```python
from build123d import *

# Parameters (mm, degrees)
ESQUISSE1_R               = 1
BOSS_EXTRU_2_DEPTH        = 6
ESQUISSE5_R               = 2
ENL_V_MAT_EXTRU_1_DEPTH   = 2
SYM_TRIE2_COPY_1_SKETCH_R = 2
SYM_TRIE2_COPY_1_DEPTH    = 2


with BuildPart() as part:
    # Esquisse1 → Boss.-Extru.2 (new body)
    with BuildSketch(Plane.XY):
        with BuildLine():
            Line((-8.804987496, 15.007737844), (-7.539903085, 12.851453671))
            ThreePointArc((-7.539903085, 12.851453671), (-5.096100136, 14.00142005), (-2.484854326, 14.691340952))
            Line((-2.484854326, 14.691340952), (-2.901776193, 17.156331045))
            ThreePointArc((-2.901776193, 17.156331045), (0, 17.4), (2.901776193, 17.156331045))
            Line((2.901776193, 17.156331045), (2.484854326, 14.691340952))
            ThreePointArc((2.484854326, 14.691340952), (5.096100136, 14.00142005), (7.539903085, 12.851453671))
            Line((7.539903085, 12.851453671), (8.804987496, 15.007737844))
            ThreePointArc((8.804987496, 15.007737844), (11.184504409, 13.32917331), (13.250766551, 11.277286278))
            Line((13.250766551, 11.277286278), (11.346920782, 9.656986526))
            ThreePointArc((11.346920782, 9.656986526), (12.903778516, 7.45), (14.036656047, 4.998228389))
            Line((14.036656047, 4.998228389), (16.391799678, 5.836857314))
            ThreePointArc((16.391799678, 5.836857314), (17.135654902, 3.021478291), (17.399575974, 0.121473929))
            Line((17.399575974, 0.121473929), (14.899636898, 0.104020778))
            ThreePointArc((14.899636898, 0.104020778), (14.67363552, -2.587357847), (13.965501643, -5.193723505))
            Line((13.965501643, -5.193723505), (16.308706617, -6.065153623))
            ThreePointArc((16.308706617, -6.065153623), (15.068842026, -8.7), (13.406930424, -11.091177422))
            Line((13.406930424, -11.091177422), (11.480647317, -9.497617447))
            ThreePointArc((11.480647317, -9.497617447), (9.577535384, -11.414062202), (7.359733812, -12.95547445))
            Line((7.359733812, -12.95547445), (8.594588479, -15.129211773))
            ThreePointArc((8.594588479, -15.129211773), (5.951150494, -16.350651602), (3.141033127, -17.114143592))
            Line((3.141033127, -17.114143592), (2.689735264, -14.655214915))
            ThreePointArc((2.689735264, -14.655214915), (0, -14.9), (-2.689735264, -14.655214915))
            Line((-2.689735264, -14.655214915), (-3.141033127, -17.114143592))
            ThreePointArc((-3.141033127, -17.114143592), (-5.951150494, -16.350651602), (-8.594588479, -15.129211773))
            Line((-8.594588479, -15.129211773), (-7.359733812, -12.95547445))
            ThreePointArc((-7.359733812, -12.95547445), (-9.577535384, -11.414062202), (-11.480647317, -9.497617447))
            Line((-11.480647317, -9.497617447), (-13.406930424, -11.091177422))
            ThreePointArc((-13.406930424, -11.091177422), (-15.068842026, -8.7), (-16.308706617, -6.065153623))
            Line((-16.308706617, -6.065153623), (-13.965501643, -5.193723505))
            ThreePointArc((-13.965501643, -5.193723505), (-14.67363552, -2.587357847), (-14.899636898, 0.104020778))
            Line((-14.899636898, 0.104020778), (-17.399575974, 0.121473929))
            ThreePointArc((-17.399575974, 0.121473929), (-17.135654902, 3.021478291), (-16.391799678, 5.836857314))
            Line((-16.391799678, 5.836857314), (-14.036656047, 4.998228389))
            ThreePointArc((-14.036656047, 4.998228389), (-12.903778516, 7.45), (-11.346920782, 9.656986526))
            Line((-11.346920782, 9.656986526), (-13.250766551, 11.277286278))
            ThreePointArc((-13.250766551, 11.277286278), (-11.184504409, 13.32917331), (-8.804987496, 15.007737844))
        make_face()
        with Locations((-6.5, -8.25)):
            Circle(ESQUISSE1_R, mode=Mode.SUBTRACT)
        with Locations((-6.5, 8.25)):
            Circle(ESQUISSE1_R, mode=Mode.SUBTRACT)
        with Locations((6.5, -8.25)):
            Circle(ESQUISSE1_R, mode=Mode.SUBTRACT)
        with Locations((6.5, 8.25)):
            Circle(ESQUISSE1_R, mode=Mode.SUBTRACT)
    extrude(amount=BOSS_EXTRU_2_DEPTH)

    # Esquisse3 → Révolution1 (revolve)
    with BuildSketch(Plane(origin=(0, 0, 0), x_dir=(1, 0, 0), z_dir=(0, 1, 0))):
        Polygon((0, -6), (-5.5, -6), (-5.5, -6.4), (-4.965, -6.4), (-4.965, -10.4), (0, -10.4), align=None)
    revolve(axis=Axis((0, 0, -3.652866049), (0, 0, 1)))

    # Esquisse4 → Enlèvement de matière-Révolution1 (revolve, cut)
    with BuildSketch(Plane(origin=(0, 0, 0), x_dir=(1, 0, 0), z_dir=(0, 1, 0)), mode=Mode.PRIVATE) as enl_vement_de_mati_re_r_volution1_sk:
        Polygon((-2.65, -6.72), (-2.65, -8.4), (-4, -8.4), (-4, -10.4), (0, -10.4), (0, 0), (-12.6, 0), (-12.6, -2.5), (-8, -2.5), (-8, -4.72), (-4, -4.72), (-4, -6.72), align=None)
    revolve(enl_vement_de_mati_re_r_volution1_sk.sketch.rotate(Axis((0, 0, 13.157502932), (0, 0, -1)), 180), axis=Axis((0, 0, 13.157502932), (0, 0, -1)), mode=Mode.SUBTRACT)

    # Esquisse5 → Enlèv. mat.-Extru.1 (cut)
    with BuildSketch(Plane.XY.offset(6)):
        with Locations((-6.5, 8.25)):
            Circle(ESQUISSE5_R)
    enl_v_mat_extru_1 = extrude(amount=-ENL_V_MAT_EXTRU_1_DEPTH, mode=Mode.SUBTRACT)

    # Symétrie1: Enlèv. mat.-Extru.1 across plane
    add(enl_v_mat_extru_1.mirror(Plane.ZX), mode=Mode.SUBTRACT)

    # Symétrie2: Enlèv. mat.-Extru.1 across plane
    add(enl_v_mat_extru_1.mirror(Plane(origin=(0, 0, 0), x_dir=(0, 0, 1), z_dir=(1, 0, 0))), mode=Mode.SUBTRACT)

    # Symétrie2 copy 1 sketch → Symétrie2 copy 1 (cut)
    with BuildSketch(Plane(origin=(0, 0, 6), x_dir=(-1, 0, 0), z_dir=(0, 0, 1))):
        with Locations((-6.5, 8.25)):
            Circle(SYM_TRIE2_COPY_1_SKETCH_R)
    extrude(amount=-SYM_TRIE2_COPY_1_DEPTH, mode=Mode.SUBTRACT)


solid = part.part
```
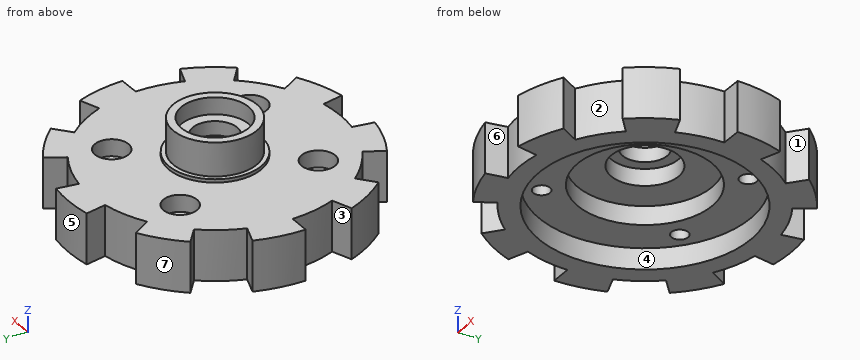
For this review, take the finished solid that the model builds, in its own axes (mm). Face numbers are marked on the shaded views. A direction names the side the tool comes from. Coordinates: 2 decimals unless noted, no trailing zeros. Order: outer loops, then holes, each group sorted by start corner. A loop starts at its lowest first (then second) coordinate and runs counter-clockwise, first axis right, second up. Notation, with made-up numbers: (-16.75, 14) - (28.25, 14) arc R20 ccw to (28.25, 22) - close; hole circle Ø2 at (13, 18.25). An arc over 180 degrees is marked (long way). Answer as a JSON object with one key per item and string values. Group by question number.
1. We need section D-D on z = 7.75. State the section outline as (x, y) points (3 decimals).
2. Clearance check with flat-ended pins moving along their axes: P1, Ø2, axis at y = 9.5, z = 7.5, coming from the -X side; P2, Ø9, axis at x = 0, y = 0, coming from the +Z side; P3, Ø3, axis at x = 7.5, y = 7.5, coming from the +Z side; P4, Ø1.2, axis at x = -6.5, y = 9, coming from the +Z side. State where each tip first meets the part, or that it passes through.
3. The part is to be moulded in two halves that separate along X. For the marked faces 5, 6 and 7, say which applies: pulls with the +X half, pulls with the -X half, needs draft (parallel to the pull), parting line crosses it, or undercut.
4. We need section C-C on z = 3.25. Give the number of separate pieces and of enclosed holes in the cut face, then the cut area to 3 significant figures.
5. For the marked faces 1, 2, 3 and 4, list the 3-axis set-ups (+Z, -Z, +X, -X, +Y, -Y) from which the entire face can be reached by the end or side of a thin tool; tool diameter is ignored.
6. We need section B-B on x = -6.5. State the section outline as (y, z) points, then the cut area to 3 significant figures.
7. For probe 1 along X at (y, z) = (8.25, 3.3); probe 2 along Y at (x, z) = (-6.5, 3.2); probe 3 along Y at (x, z) = (13, 5.5), list the stretches that pass through material, from the lowest coordinate up.
Final values:
{
 "1": {"outline": "circle Ø9.93 at (0, 0); hole circle Ø5.3 at (0, 0)"},
 "2": {"P1": "through", "P2": "z = 10.4", "P3": "z = 6", "P4": "z = 4"},
 "3": {"face 5": "parting line crosses it", "face 6": "undercut", "face 7": "pulls with the -X half"},
 "4": {"separate pieces": "1", "enclosed holes": "5", "area": "606 mm²"},
 "5": {"face 1": "+Z, -Z, +X", "face 2": "+Z, -Z", "face 3": "+Z, -Z, -X", "face 4": "-Z"},
 "6": {"outline": "(-16.14, 0) - (-10.79, 0) - (-10.79, 2.5) - (-9.25, 2.5) - (-9.25, 4) - (-10.25, 4) - (-10.25, 6) - (-16.14, 6) - close; (-7.25, 2.5) - (-4.66, 2.5) - (-4.66, 4.72) - (4.66, 4.72) - (4.66, 2.5) - (7.25, 2.5) - (7.25, 4) - (6.25, 4) - (6.25, 6) - (-6.25, 6) - (-6.25, 4) - (-7.25, 4) - close; (9.25, 2.5) - (10.79, 2.5) - (10.79, 0) - (13.41, 0) - (13.41, 6) - (10.25, 6) - (10.25, 4) - (9.25, 4) - close", "area": "80.6 mm²"},
 "7": {"probe 1": "-12.41 to -7.5, -5.5 to 5.5, 7.5 to 12.41", "probe 2": "-16.14 to -9.25, -7.25 to -4.66, 4.66 to 7.25, 9.25 to 13.41", "probe 3": "-10.75 to 7.28, 11.06 to 11.57"}
}
